Geometry check sheet. Reference: the model listing, model coordinates, mm. A direction names the side the tool comes from. Give positions to 0.01 mm unless a question says otherwise; leave off trailing zeros. Write each loop counter-clockwise with the first axis right and the second up, starting at its lowest first coordinate (ties: lowest second). Pieces come first, ordered by that corner, then holes. Notation, with made-up numbers: (60.5, 37) -> (75.5, 37) arc R19 ccw to (75.5, 73) -> close; hole circle Ø3 at (57, 24.25). An arc over 180 degrees is marked (long way). One line per item, written item: value.
from build123d import *

# Parameters (mm, degrees)
F0_W     = 6
F0_H     = 19
F1_DEPTH = 3
F2_W     = 6
F2_H     = 2
F3_DEPTH = 3
F4_R     = 1.75
F5_DEPTH = 3
F6_W     = 19
F6_H     = 12
F7_DEPTH = 3
F8_R     = 1.5
F9_DEPTH = 3
F10_R    = 5
F11_R    = 3


with BuildPart() as f1:
    # F0 (on Top) → F1 (new body)
    with BuildSketch(Plane.XY):
        with Locations((3, 0)):
            Rectangle(F0_W, F0_H)
    extrude(amount=F1_DEPTH)

    # F2 (on face) → F3 (join)
    with BuildSketch(Plane(origin=(0, 0, 0), x_dir=(1, 0, 0), z_dir=(0, 0, -1))):
        with Locations((3, 8.5)):
            Rectangle(F2_W, F2_H)
        with Locations((3, -8.5)):
            Rectangle(F2_W, F2_H)
    extrude(amount=F3_DEPTH)

    # F4 (on face) → F5 (cut)
    with BuildSketch(Plane.XY.offset(3)):
        with Locations((3, 0)):
            Circle(F4_R)
    extrude(amount=-F5_DEPTH, mode=Mode.SUBTRACT)

    # F6 (on face) → F7 (join)
    with BuildSketch(Plane(origin=(0, 0, 0), x_dir=(0, -1, 0), z_dir=(-1, 0, 0))):
        with Locations((0, 9)):
            Rectangle(F6_W, F6_H)
        Polygon((-9.5, 3), (-9.5, 0), (-7.5, 0), (7.5, 0), (9.5, 0), (9.5, 3), align=None)
    extrude(amount=F7_DEPTH)

    # F8 (on face) → F9 (cut)
    with BuildSketch(Plane.YZ):
        with Locations((0, 11.2423589453)):
            Circle(F8_R)
    extrude(amount=-F9_DEPTH, mode=Mode.SUBTRACT)

    # F10
    f10_edges = [f1.edges().sort_by_distance(p)[0] for p in [
        (-1.5, -9.5, 15),
        (-1.5, 9.5, 15),
    ]]
    fillet(f10_edges, radius=F10_R)

    # F11
    f11_edges = [f1.edges().sort_by_distance(p)[0] for p in [
        (3, -9.5, 3),
        (3, 9.5, 3),
    ]]
    fillet(f11_edges, radius=F11_R)


solid = f1.part
1) Sectioned sample at B-B on y = 0. Record the cut outline in (x, z).
Verdict:
outline: (-3, 0) -> (1.25, 0) -> (1.25, 3) -> (0, 3) -> (0, 9.74) -> (-3, 9.74) -> close; (-3, 12.74) -> (0, 12.74) -> (0, 15) -> (-3, 15) -> close; (4.75, 0) -> (6, 0) -> (6, 3) -> (4.75, 3) -> close
2) Sectioned sample at A-A on x = 3. Record the cut outline in (y, z), plus the area to 3 significant figures.
Verdict:
outline: (-9.5, -3) -> (-7.5, -3) -> (-7.5, 0) -> (-1.75, 0) -> (-1.75, 3) -> (-6.5, 3) arc R3 ccw to (-9.5, 0) -> close; (1.75, 0) -> (7.5, 0) -> (7.5, -3) -> (9.5, -3) -> (9.5, 0) arc R3 ccw to (6.5, 3) -> (1.75, 3) -> close
area: 54.6 mm^2
3) Mould release check, pull along Y, two halves, no side actions. Record for faces 4 (the flat face through (3, 7.5, -1)), 5 (the flat face through (6, 0, 1)), 6 (the flat face through (3, -7.5, -1)), 7 (the cylindrical face through (3.04, -8.6, 2.14)): released by +Y, released by -Y, zero draft, split by the parting line, or undercut.
Verdict:
face 4: undercut
face 5: zero draft
face 6: undercut
face 7: released by -Y
4) Depth check by flat-ended pin: pin 1 Ø5 at (x, y) = (4, -6) entering from +Z; pin 2 Ø4 at (y, z) = (5, 11) entering from +X; pin 3 Ø2 at (y, z) = (8, -2) entering from -X; pin 4 Ø2 at (x, y) = (3, 0) entering from -Z. Enter the tip coordinate at first touch or a pass-through.
Verdict:
pin 1: z = 3
pin 2: x = 0
pin 3: x = 0
pin 4: through
5) Sectioned sample at C-C on x = 0.5. Record the cut outline in (y, z), plus the area to 3 significant figures.
Verdict:
outline: (-9.5, -3) -> (-7.5, -3) -> (-7.5, 0) -> (7.5, 0) -> (7.5, -3) -> (9.5, -3) -> (9.5, 0) arc R3 ccw to (6.5, 3) -> (-6.5, 3) arc R3 ccw to (-9.5, 0) -> close
area: 65.1 mm^2
6) Sectioned sample at D-D on z = 2.5. Record the cut outline in (x, y), plus the area to 3 significant figures.
Verdict:
outline: (-3, -9.5) -> (0, -9.5) -> (0, -8.16) -> (6, -8.16) -> (6, 8.16) -> (0, 8.16) -> (0, 9.5) -> (-3, 9.5) -> close; hole circle Ø3.5 at (3, 0)
area: 145 mm^2
7) Tool access check on faces 1 (the cylindrical face through (3.04, 8.64, 2.1)), 2 (the cylindrical face through (4.669, 0.526, 1.521)), 3 (the flat face through (0, 9, -1)). Record the directions out of +Z, -Z, +X, -X, +Y, -Y that give a thin tool (end or side, any length) a straight path to the whole face; none if there is none.
Verdict:
face 1: +Z, +X, +Y
face 2: +Z, -Z
face 3: -Z, -X, +Y, -Y
8) Scan lines: probe 1 along Z at (x, y) = (-1.3, 0); probe 2 along Z at (x, y) = (4, 4.25); probe 3 along X at (y, z) = (-4, 4). Record each from-to range of solid material in increasing order.
Verdict:
probe 1: 0 to 9.74, 12.74 to 15
probe 2: 0 to 3
probe 3: -3 to 0
